The listing builds one solid part. Answer for the finished solid, in the listing's coordinates (mm). Face numbers are marked on the shaded views. A direction names the side the tool comes from. Coordinates: 2 decimals unless noted, no trailing zeros. Loops run counter-clockwise (first coordinate to the right, second up) from the corner with the lowest first, then second, coordinate; pieces in that order, holes last. Notation, with made-up numbers: M -26.75,-23.75 L -15.75,-23.75 A20 cw -15.75,-10.75 Z; hole C 53.25,72 d8. An arc over 180 degrees is marked long. Return JSON: item names as keys, results as strings. Group by question number.
1. Which of the six approach directions +Z, -Z, +X, -X, +Y, -Y give full straight-line access (tool end or side, diameter ignored) to the marked faces 1, 2, 3 and 4?
2. Given P1, Ø2, axis at x = 8.5, z = 35.5, coming from the +Y side; P2, Ø10, axis at y = 5, z = 52.5, coming from the +X side; P3, Ø1, axis at x = 5, z = 65.5, coming from the -Y side; P4, Ø8, axis at x = -11, y = -1.5, coming from the +Z side, each flat-ended and moving along its own axis, determine where each tip first touches the part or whether it passes through.
3. The mould has two halves that part along Y. Classify the marked faces 5, 6, 7 and 8: pulls with the +Y half, pulls with the -Y half, needs draft (parallel to the pull), parting line crosses it, or undercut.
4. Section D-D (x = 8) is taken. Write down the section's boundary in (y, z), then the cut area to 3 significant figures.
5. Straight lines are drawn through the part: L1, parallel to Y at x = 1.4, z = 50; L2, parallel to Z at x = -0.5, y = 15; L3, parallel to Y at x = 12, z = 37.5. For each, find the intervals that lie inside material, in ascending order. Write a range as from..to.
6. Section C-C (x = -9) is taken. Write down the section's boundary in (y, z), then the cut area to 3 significant figures.
7. Section A-A (y = 0) is taken. Count the separate pieces of the cut face and the enclosed holes in it, then the cut area to 3 significant figures.
```python
from build123d import *

# Parameters (mm, degrees)
F3_D     = 10
F3_DEPTH = 20.001
F4_D     = 10


with BuildPart() as f1:
    # F0 (on Front) → F1 (revolve)
    with BuildSketch(Plane.XZ):
        Polygon((-20, 18), (-20, 0), (-13, 0), (-6, 12.5), (0, 12.5), (6, 12.5), (13, 0), (20, 0), (20, 18), (6, 22), (0, 22), (-6, 22), align=None)
        Polygon((-6, 33), (-6, 22), (0, 22), (6, 22), (6, 33), (0, 33), align=None)
        Polygon((-15, 33), (-6, 33), (0, 33), (6, 33), (15, 33), (15, 40), (0, 40), (-15, 40), align=None)
    revolve(axis=Axis((-4.1045919061, 0, 50), (1, 0, 0)))

    # F3 (through all, one way)
    with BuildSketch(Plane.YZ):
        with Locations((15.9099025767, 65.9099025767), (0, 72.5), (-15.9099025767, 65.9099025767), (-22.5, 50), (-15.9099025767, 34.0900974233), (0, 27.5), (15.9099025767, 34.0900974233), (22.5, 50)):
            Circle(F3_D / 2)
    extrude(amount=-F3_DEPTH, mode=Mode.SUBTRACT)

    # F4 (through all)
    with Locations(Plane(origin=(0, 0, 0), x_dir=(0, 1, 0), z_dir=(-1, 0, 0))):
        with Locations((0, -72.5), (15.9099025767, -65.9099025767), (22.5, -50), (15.9099025767, -34.0900974233), (0, -27.5), (-15.9099025767, -34.0900974233), (-22.5, -50), (-15.9099025767, -65.9099025767)):
            Hole(F4_D / 2)


solid = f1.part
```
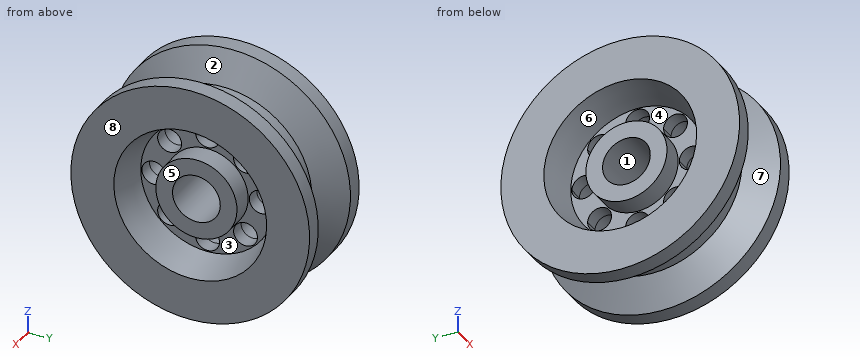
Worked out:
{
 "1": {"face 1": "+X, -X", "face 2": "none", "face 3": "+X", "face 4": "-X"},
 "2": {"P1": "y = 41.31", "P2": "x = 15", "P3": "y = -34.37", "P4": "z = 100"},
 "3": {"face 5": "undercut", "face 6": "undercut", "face 7": "parting line crosses it", "face 8": "needs draft"},
 "4": {"outline": "C 0,50 d82.14; C 0,50 d34; hole C 0,50 d57.14; hole C 0,50 d20", "area": "3,330 mm^2"},
 "5": {"L1": "-37.5..-27.5, -17.5..-10, 10..17.5, 27.5..37.5", "L2": "15.63..29.17, 39.01..60.99, 70.83..84.37", "L3": "-46.57..-26.96, -11.52..11.52, 26.96..46.57"},
 "6": {"outline": "C 0,50 d85.71; C 0,50 d34; hole C 0,50 d57.71; hole C 0,50 d20", "area": "3,750 mm^2"},
 "7": {"separate pieces": "4", "enclosed holes": "0", "area": "1,620 mm^2"}
}
